from build123d import *

# Parameters (mm, degrees)
F0_R     = 3
F1_DEPTH = 10


with BuildPart() as f1:
    # F0 (on Top) → F1 (new body)
    with BuildSketch(Plane.XY):
        with BuildLine():
            ThreePointArc((0.600467, 390.036187), (4.990945, 395.300778), (0, 400))
            ThreePointArc((0, 400), (-199.565588, 213.17483), (-26.292427, 1.735761))
            Line((-26.292427, 1.735761), (26.292427, -5.237677))
            ThreePointArc((26.292427, -5.237677), (160.690327, -196.187456), (-0.600467, -365.036187))
            ThreePointArc((-0.600467, -365.036187), (-4.990945, -370.300778), (0, -375))
            ThreePointArc((0, -375), (199.565588, -188.17483), (26.292427, 23.264239))
            Line((26.292427, 23.264239), (-26.292427, 30.237677))
            ThreePointArc((-26.292427, 30.237677), (-160.690327, 221.187456), (0.600467, 390.036187))
        make_face()
        with Locations((0, 12.5)):
            Circle(F0_R, mode=Mode.SUBTRACT)
    extrude(amount=F1_DEPTH)


solid = f1.part
The model under review builds one solid part; all positions refer to its coordinate system, in mm. Coordinates: 2 decimals unless noted, no trailing zeros. Write each loop counter-clockwise with the first axis right and the second up, starting at its lowest first coordinate (ties: lowest second). Pieces come first, ordered by that corner, then holes. Notation, with made-up numbers: (34.25, 13) - (84.25, 13) arc R7 cw to (84.25, 21) - close; hole circle Ø11 at (77, 80). An arc over 180 degrees is marked (long way). Answer as a JSON object with one key per item and string values. Group by question number.
1. Clearance check with flat-ended pins moving along their axes: pin 1 Ø5 at (y, z) = (-173, 3.5) entering from -X; pin 2 Ø6 at (y, z) = (322, 5) entering from +X; pin 3 Ø2 at (x, z) = (-101, 2) entering from +Y. State where each tip first meets the part, or that it passes through.
2. Add section C-C (x = 152). Give the boundary of the cut face in (y, z).
3. To check wall thickness, follow probe 1 along Y at (x, z) = (33, 3); probe 2 along X at (y, z) = (200, 9.75); probe 3 along Y at (x, z) = (-75, 7). State the ranges of each line that lie inside material, in increasing order.
4. Add section A-A (z = 8). Give the boundary of the cut face in (x, y), plus the area to 3 significant figures.
5. Add section B-B (x = -52.5). Give the boundary of the cut face in (y, z), plus the area to 3 significant figures.
6. Add section D-D (y = -263.5). Give the boundary of the cut face in (x, z), plus the area to 3 significant figures.
Findings:
{
 "1": {"pin 1": "x = 160.81", "pin 2": "x = -118.75", "pin 3": "y = 373.21"},
 "2": {"outline": "(-304.98, 0) - (-239.92, 0) - (-239.92, 10) - (-304.98, 10) - close; (-125.04, 0) - (-45.02, 0) - (-45.02, 10) - (-125.04, 10) - close"},
 "3": {"probe 1": "-372.26 to -357.73, -7.23 to 22.26", "probe 2": "-200 to -161.05", "probe 3": "14.6 to 51.69, 363.28 to 385.4"},
 "4": {"outline": "(-26.29, 1.74) - (26.29, -5.24) arc R183.89 cw to (-0.6, -365.04) arc R5 ccw to (0, -375) arc R200 ccw to (26.29, 23.26) - (-26.29, 30.24) arc R183.89 cw to (0.6, 390.04) arc R5 ccw to (0, 400) arc R200 ccw to start; hole circle Ø6 at (0, 12.5)", "area": "36,200 mm²"},
 "5": {"outline": "(7.01, 0) - (39.67, 0) - (39.67, 10) - (7.01, 10) - close; (375.29, 0) - (392.99, 0) - (392.99, 10) - (375.29, 10) - close", "area": "503 mm²"},
 "6": {"outline": "(142.39, 0) - (179.35, 0) - (179.35, 10) - (142.39, 10) - close", "area": "370 mm²"}
}
